Build history of the part. All positions in model axes, mm. Face numbers are marked on the shaded views. A direction names the side the tool comes from. Give positions to 0.01 mm unless a question says otherwise; leave off trailing zeros. Write each loop counter-clockwise with the first axis right and the second up, starting at its lowest first coordinate (ties: lowest second). Pieces come first, ordered by that corner, then holes. Notation, with made-up numbers: (18.5, 68.5) -> (59.5, 68.5) arc R14 cw to (59.5, 84.5) -> close; hole circle Ø3 at (18.25, 23). An arc over 180 degrees is marked (long way). Write item = value, one per line. Start each with the question number.
Q1. Wall check: line 1 (X direction, y = 5.75, z = 3); line 2 (Y direction, x = 2.5, z = 3.5). Give the ranges that are in metal, low to high.
Q2. Saw through at C-C, the plane x = -2. List the corners of the cut face in (y, z), then the cut area to 3 significant figures.
Q3. Saw through at A-A, the plane y = 5.25. List the corners of the cut face in (x, z), then the cut area to 3 significant figures.
Q4. Mould opens along X. For the marked faces 3, 4 and 5 say: pulls with the +X half, pulls with the -X half, needs draft (parallel to the pull), parting line crosses it, or undercut.
Q5. Saw through at B-B, the plane z = 7. List the corners of the cut face in (x, y), then the cut area to 3 significant figures.
Q6. Tool access for the marked faces 1 and 2: list every direction of +Z, -Z, +X, -X, +Y, -Y with a clear straight run to the whole face (end or side of a thin tool).
Q7. Drop a flat-ended pin along its axis: P1, Ø3, axis at x = 0.5, z = 3, coming from the +Y side. Give the stop position or say it passes through.
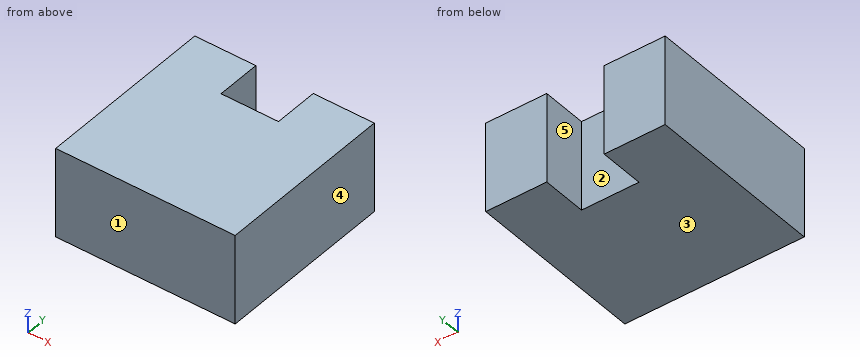
from build123d import *

# Parameters (mm, degrees)
SKETCH_1_W          = 20
SKETCH_1_H          = 20
EXTRUDE_1_DEPTH     = 10
CUT_EXTRUDE_1_DEPTH = 10


with BuildPart() as part:
    # 草图1 → 凸台-拉伸1 (new body)
    with BuildSketch(Plane.XY):
        Rectangle(SKETCH_1_W, SKETCH_1_H)
    extrude(amount=EXTRUDE_1_DEPTH)

    # 草图2 → 切除-拉伸1 (cut)
    with BuildSketch(Plane.XY.offset(10)):
        Polygon((0, 10), (3.2, 10), (3.2, 5), (-3.2, 5), (-3.2, 10), align=None)
    extrude(amount=-CUT_EXTRUDE_1_DEPTH, mode=Mode.SUBTRACT)


solid = part.part
Report:
q1.line_1 = -10 to -3.2, 3.2 to 10
q1.line_2 = -10 to 5
q2.outline = (-10, 0) -> (5, 0) -> (5, 10) -> (-10, 10) -> close
q2.area = 150 mm2
q3.outline = (-10, 0) -> (-3.2, 0) -> (-3.2, 10) -> (-10, 10) -> close; (3.2, 0) -> (10, 0) -> (10, 10) -> (3.2, 10) -> close
q3.area = 136 mm2
q4.face_3 = needs draft
q4.face_4 = pulls with the +X half
q4.face_5 = undercut
q5.outline = (-10, -10) -> (10, -10) -> (10, 10) -> (3.2, 10) -> (3.2, 5) -> (-3.2, 5) -> (-3.2, 10) -> (-10, 10) -> close
q5.area = 368 mm2
q6.face_1 = +Z, -Z, +X, -X, -Y
q6.face_2 = +Z, -Z, +Y
q7.P1 = 5
